from build123d import *

# Parameters (mm, degrees)
F0_R          = 21.59
F1_DEPTH      = 76.2
F2_R          = 33.897036
F2_R_2        = 21.59
F3_DEPTH      = 7.62
F4_R          = 15.833015
F5_DEPTH      = 83.821
F6_R          = 44.45
F7_DEPTH      = 25.4
F7_DEPTH_BACK = 38.4834


with BuildPart() as f1:
    # F0 (on Front) → F1 (new body)
    with BuildSketch(Plane.XZ):
        Circle(F0_R)
    extrude(amount=F1_DEPTH)

    # F2 (on face) → F3 (join)
    with BuildSketch(Plane.XZ.offset(76.2)):
        Circle(F2_R)
        Circle(F2_R_2, mode=Mode.SUBTRACT)
        Circle(F2_R_2)
    extrude(amount=F3_DEPTH)

    # F4 (on face) → F5 (cut, through all)
    with BuildSketch(Plane.XZ.offset(83.82)):
        Circle(F4_R)
    extrude(amount=-F5_DEPTH, mode=Mode.SUBTRACT)

    # F6 (on Top) → F7 (cut, two sides)
    with BuildSketch(Plane.XY) as f7_sk:
        with Locations((0, 26.801758)):
            Circle(F6_R)
    extrude(amount=F7_DEPTH, mode=Mode.SUBTRACT)
    extrude(f7_sk.sketch, amount=-F7_DEPTH_BACK, mode=Mode.SUBTRACT)


solid = f1.part
The listing builds one solid part. Answer for the finished solid, in the listing's coordinates (mm). A direction names the side the tool comes from. Give positions to 0.01 mm unless a question says otherwise; leave off trailing zeros. Write each loop counter-clockwise with the first axis right and the second up, starting at its lowest first coordinate (ties: lowest second). Pieces come first, ordered by that corner, then holes. Notation, with made-up numbers: (38.5, 32.5) - (91.5, 32.5) arc R12 ccw to (91.5, 55.5) - close; hole circle Ø4 at (17.25, -35.75). An arc over 180 degrees is marked (long way). One line per question, with ' | ' between items. Start each with the question number.
1. Section B-B, the plane z = 0 is taken. Determine the outline of the cut face in (x, y).
2. Straight lines are drawn through the part: line 1 (X direction, y = -55, z = 0); line 2 (Y direction, x = 7, z = 29). For each, find the intervals that lie inside material, in ascending order.
3. Given P1, Ø2, axis at x = -9.5, z = -25.5, coming from the +Y side; P2, Ø8, axis at x = 15, y = -50, coming from the +Z side; P3, Ø6, axis at x = -21.5, y = -48, coming from the +Z side, each flat-ended and moving along its own axis, determine where each tip first touches the part or whether it passes through.
4. Section D-D, the plane z = 20 is taken. Determine the outline of the cut face in (x, y), then the cut area to 3 significant figures.
5. Determine the mould class of faces 1 (the face through (15, -83.82, -7)), 2 (the face through (-21.57, -43.68, 0.95)), 3 (the face through (-12.565, -49.76, -9.634)) for opening direction Z: +Z half, -Z half, draft (parallel to the pull), parting line (faces both ways), or undercut.
6. Section C-C, the plane y = -73 is taken. Determine the outline of the cut face in (x, z), then the cut area to 3 significant figures.
7. Section A-A, the plane x = 0 is taken. Determine the outline of the cut face in (y, z), then the cut area to 3 significant figures.
8. For faces 4 (the face through (0, -76.2, -22)), 5 (the face through (9.832, -16.547, 12.696)), determine the directions among +Z, -Z, +X, -X, +Y, -Y from which every point of the face is accessible in a straight line to the end or side of a thin tool.
Result:
1) outline: (-33.9, -83.82) - (-15.83, -83.82) - (-15.83, -14.73) arc R44.45 cw to (-21.59, -12.05) - (-21.59, -76.2) - (-33.9, -76.2) - close; (15.83, -83.82) - (33.9, -83.82) - (33.9, -76.2) - (21.59, -76.2) - (21.59, -12.05) arc R44.45 cw to (15.83, -14.73) - close
2) line 1: x = -21.59 to -15.83, 15.83 to 21.59 | line 2: y = -83.82 to -76.2
3) P1: stops at y = -76.2 | P2: stops at z = 18.58 | P3: stops at z = 11.13
4) outline: (-27.37, -83.82) - (27.37, -83.82) - (27.37, -76.2) - (8.13, -76.2) - (8.13, -16.9) arc R44.45 cw to (-8.13, -16.9) - (-8.13, -76.2) - (-27.37, -76.2) - close | area: 1,370 mm2
5) face 1: draft | face 2: parting line | face 3: undercut
6) outline: circle Ø43.18 at (0, 0); hole circle Ø31.67 at (0, 0) | area: 677 mm2
7) outline: (-83.82, -33.9) - (-76.2, -33.9) - (-76.2, -21.59) - (-17.65, -21.59) - (-17.65, -15.83) - (-83.82, -15.83) - close; (-83.82, 15.83) - (-17.65, 15.83) - (-17.65, 21.59) - (-76.2, 21.59) - (-76.2, 33.9) - (-83.82, 33.9) - close | area: 949 mm2
8) face 4: +Y | face 5: +Z, -Z, +Y
